For this review, take the finished solid that the model builds, in its own axes (mm). Coordinates: 2 decimals unless noted, no trailing zeros. Loops run counter-clockwise (first coordinate to the right, second up) from the corner with the lowest first, then second, coordinate; pieces in that order, holes last. Notation, with made-up numbers: (-23.5, 61) -> (-19.5, 61) arc R15 ccw to (-19.5, 74) -> close; hole circle Ø5 at (27, 30). An arc over 180 degrees is marked (long way). Use a Markdown table: item, result.
from build123d import *

# Parameters (mm, degrees)
F1_DEPTH = 0.4


with BuildPart() as f1:
    # F0 (on Top) → F1 (new body)
    with BuildSketch(Plane.XY):
        with BuildLine():
            Line((-21.9038240612, -39.2802841961), (0, -37.8296988058))
            Line((0, -37.8296988058), (0, 1.5558084287))
            Line((0, 1.5558084287), (-49.4176484644, 1.5558084287))
            Line((-49.4176484644, 1.5558084287), (-49.4176484644, -39.5778827369))
            Line((-49.4176484644, -39.5778827369), (-44, -39.5778827369))
            add(Edge.make_bspline(
                [(-44, -39.5778827369), (-41.9009812176, -31.3107147813), (-39.967373394, -23.2768925028), (-35.7254609829, -17.6712276554), (-35.032177344, -16.9143821545)],
                knots=[0, 0, 0, 0, 0.545331607, 0.6402959588, 0.6402959588, 0.6402959588, 0.6402959588], degree=3))
            Line((-35.032177344, -16.9143821545), (-35.032177344, -5.9383278713))
            Line((-35.032177344, -5.9383278713), (-23.665998131, -5.9383278713))
            Line((-23.665998131, -5.9383278713), (-23.665998131, -12.6714743674))
            Line((-23.665998131, -12.6714743674), (-21.9038240612, -39.2802841961))
        make_face()
        with BuildLine():
            Line((21.9038240612, -39.2802841961), (23.665998131, -12.6714743674))
            add(Edge.make_bspline(
                [(44, -39.5778827369), (41.9009812176, -31.3107147813), (38.8811154869, -18.7636696725), (30.2309490173, -12.1392643454), (23.665998131, -12.6714743674)],
                knots=[0, 0, 0, 0, 0.545331607, 1, 1, 1, 1], degree=3))
            Line((44, -39.5778827369), (49.4176484644, -39.5778827369))
            Line((49.4176484644, -39.5778827369), (49.4176484644, 1.5558084287))
            Line((49.4176484644, 1.5558084287), (0, 1.5558084287))
            Line((0, 1.5558084287), (0, -37.8296988058))
            Line((0, -37.8296988058), (21.9038240612, -39.2802841961))
        make_face()
    extrude(amount=F1_DEPTH)


solid = f1.part
(1) For line 1 along X through (y, z) = (-11, 0.35); line 2 along X through (y, z) = (-29.5, 0.1); line 3 along X through (y, z) = (-20, 0.2), list the stretches that pass through material, from the lowest coordinate up.
Found:
| item | result |
|---|---|
| line 1 | x = -49.42 to -35.03, -23.67 to 49.42 |
| line 2 | x = -49.42 to -41.3, -22.55 to 22.55, 41.3 to 49.42 |
| line 3 | x = -49.42 to -37.32, -23.18 to 23.18, 37.32 to 49.42 |
(2) Mouldability with a two-part tool opening along X and no side actions: class faces 1 (the face through (22.773, -26.162, 0.197)), 2 (the face through (-1, -19, 0.4)), 3 (the face through (-22.797, -25.79, 0.197)) as pulls with the +X half, pulls with the -X half, needs draft (parallel to the pull), parting line crosses it, or undercut.
Found:
| item | result |
|---|---|
| face 1 | undercut |
| face 2 | needs draft |
| face 3 | undercut |
(3) Take a section at B-B on x = -15. Write out the cut boundary in (y, z), plus the area to 3 significant figures.
Found:
| item | result |
|---|---|
| outline | (-38.82, 0) -> (1.56, 0) -> (1.56, 0.4) -> (-38.82, 0.4) -> close |
| area | 16.2 mm^2 |
(4) Take a section at A-A on y = -21.5. State how many separate pieces and enclosed holes the cut face has, plus the area to 3 significant figures.
Found:
| item | result |
|---|---|
| separate pieces | 3 |
| enclosed holes | 0 |
| area | 27.5 mm^2 |
(5) Take a section at D-D on x = 4. Write out the cut boundary in (y, z).
Found:
| item | result |
|---|---|
| outline | (-38.09, 0) -> (1.56, 0) -> (1.56, 0.4) -> (-38.09, 0.4) -> close |
(6) For pin 1 Ø1 at (x, y) = (38.5, -16.5) entering from -Z, flat-tipped, find the tip position at first contact; note if it passes through.
Found:
| item | result |
|---|---|
| pin 1 | stops at z = 0 |
